from build123d import *

# Parameters (mm, degrees)
SKETCH1_W               = 40
SKETCH1_H               = 95
BOSS_EXTRUDE1_DEPTH     = 3
SKETCH2_W               = 2.5
SKETCH2_H               = 2.5
BOSS_EXTRUDE2_DEPTH     = 3
CUT_EXTRUDE1_DEPTH      = 104.121287812
CUT_EXTRUDE1_DEPTH_BACK = 104.121287812
SKETCH3_W               = 22
SKETCH3_H               = 24
SKETCH3_W_2             = 5
SKETCH3_H_2             = 23
SKETCH3_W_3             = 11
SKETCH3_H_3             = 10


with BuildPart() as part:
    # Sketch1 → Boss-Extrude1 (new body)
    with BuildSketch(Plane(origin=(0, 0, 0), x_dir=(1, 0, 0), z_dir=(0, 1, 0))):
        with Locations((-20, 47.5)):
            Rectangle(SKETCH1_W, SKETCH1_H)
    extrude(amount=BOSS_EXTRUDE1_DEPTH)

    # Sketch2 → Boss-Extrude2 (add)
    with BuildSketch(Plane(origin=(0, 3, 0), x_dir=(1, 0, 0), z_dir=(0, 1, 0))):
        with Locations((-3.5, 3.5)):
            Rectangle(SKETCH2_W, SKETCH2_H)
        with Locations((-36.5, 3.5)):
            Rectangle(SKETCH2_W, SKETCH2_H)
        with Locations((-36.5, 91.5)):
            Rectangle(SKETCH2_W, SKETCH2_H)
    extrude(amount=BOSS_EXTRUDE2_DEPTH)

    # Sketch3 → Cut-Extrude1 (cut, two sides: drawn at the far end of the back side and taken through both)
    with BuildSketch(Plane(origin=(0, 3, 0), x_dir=(1, 0, 0), z_dir=(0, 1, 0)).offset(-CUT_EXTRUDE1_DEPTH_BACK)):
        with Locations((-16, 83)):
            Rectangle(SKETCH3_W, SKETCH3_H)
        with Locations((-2.5, 57.5)):
            Rectangle(SKETCH3_W_2, SKETCH3_H_2)
        with Locations((-5.5, 32)):
            Rectangle(SKETCH3_W_3, SKETCH3_H_3)
        with Locations((-25.5, 32)):
            Rectangle(SKETCH3_W_3, SKETCH3_H_3)
    extrude(amount=CUT_EXTRUDE1_DEPTH + CUT_EXTRUDE1_DEPTH_BACK, mode=Mode.SUBTRACT)


solid = part.part
Verification items for the finished model (mm, model axes). A direction names the side the tool comes from. Round coordinates to 2 decimals unless told otherwise and drop trailing zeros. Write each loop counter-clockwise with the first axis right and the second up, starting at its lowest first coordinate (ties: lowest second). Pieces come first, ordered by that corner, then holes.
(1) Section check D-D (z = -23). Enter the section's corners in (x, y), plus the area to 3 significant figures.
Returned:
outline: (-40, 0) - (0, 0) - (0, 3) - (-40, 3) - close
area: 120 mm2
(2) Depth check by flat-ended pin: pin 1 Ø2 at (y, z) = (4.5, -91) entering from +X; pin 2 Ø1.2 at (y, z) = (4, -3.5) entering from -X; pin 3 Ø6 at (x, z) = (-22.5, -42.5) entering from +Y; pin 4 Ø1.5 at (x, y) = (-22.5, 5.5) entering from -Z. Enter the tip coordinate at first touch or a pass-through.
Returned:
pin 1: stops at x = -35.25
pin 2: stops at x = -37.75
pin 3: stops at y = 3
pin 4: passes through
(3) Section check C-C (y = 1.35). Enter the section's corners in (x, z), plus the area to 3 significant figures.
Returned:
outline: (-40, -95) - (-27, -95) - (-27, -71) - (-5, -71) - (-5, -95) - (0, -95) - (0, -69) - (-5, -69) - (-5, -46) - (0, -46) - (0, -37) - (-11, -37) - (-11, -27) - (0, -27) - (0, 0) - (-40, 0) - close; hole (-31, -37) - (-20, -37) - (-20, -27) - (-31, -27) - close
area: 2,940 mm2
(4) Access from +Z, -Z, +X, -X, +Y, -Y to the whole of each face (thin tool, end or side, straight path). Record for faces 1 (the flat face through (-35.25, 4, -91)), 2 (the flat face through (-4.75, 4, -3)), 3 (the flat face through (-37.75, 4, -91)), 4 (the flat face through (-26, 1, -27)), 5 (the flat face through (-11, 1, -32)).
Returned:
face 1: +Z, -Z, +X, +Y
face 2: +Z, -Z, +Y
face 3: +Z, -Z, -X, +Y
face 4: +Y, -Y
face 5: +X, +Y, -Y
(5) Mould release check, pull along Z, two halves, no side actions. Record for faces 6 (the flat face through (-37, 6, -4)), 7 (the flat face through (-34, 1, -95)), 8 (the flat face through (-20, 1, -32)): pulls with the +Z half, pulls with the -Z half, needs draft (parallel to the pull), parting line crosses it, or undercut.
Returned:
face 6: needs draft
face 7: pulls with the -Z half
face 8: undercut
(6) Section check A-A (z = -32.5). Enter the section's corners in (x, y), plus the area to 3 significant figures.
Returned:
outline: (-40, 0) - (-31, 0) - (-31, 3) - (-40, 3) - close; (-20, 0) - (-11, 0) - (-11, 3) - (-20, 3) - close
area: 54.0 mm2
(7) Section check B-B (x = -9). Enter the section's corners in (y, z).
Returned:
outline: (0, -71) - (3, -71) - (3, -37) - (0, -37) - close; (0, -27) - (3, -27) - (3, 0) - (0, 0) - close
(8) Material ranges on line 1 (X direction, y = 2.5, z = -31); line 2 (X direction, y = 2.9, z = -78.5); line 3 (Z direction, x = -30, y = 2.1), recorded low to high.
Returned:
line 1: x = -40 to -31, -20 to -11
line 2: x = -40 to -27, -5 to 0
line 3: z = -95 to -37, -27 to 0
